```python
from build123d import *

# Parameters (mm, degrees)
SKETCH1_W           = 12.45
SKETCH1_H           = 21.45
BOSS_EXTRUDE1_DEPTH = 18
SKETCH2_W           = 10
SKETCH2_H           = 3
BOSS_EXTRUDE2_DEPTH = 18
SKETCH4_W           = 7
SKETCH4_H           = 8.185466936
SKETCH4_H_2         = 9.121133548
SKETCH4_H_3         = 13.415591142
SKETCH4_H_4         = 10.11507115
SKETCH4_H_5         = 8.575799248
CUT_EXTRUDE2_DEPTH  = 6
FILLET3_R           = 3.5
FILLET4_R           = 2
SKETCH5_R           = 1.6
CUT_EXTRUDE3_DEPTH  = 105.163684291
CUT_EXTRUDE4_DEPTH  = 105.163684291
SKETCH10_W          = 7.3675
SKETCH10_H          = 18
SKETCH10_R          = 1.6
BOSS_EXTRUDE4_DEPTH = 21.45
FILLET6_R           = 3
SKETCH11_W          = 114.139507882
SKETCH11_H          = 1
CUT_EXTRUDE5_DEPTH  = 97.285728563
CHAMFER1_SIZE       = 1
CHAMFER2_SIZE       = 1
FILLET7_R           = 1
FILLET8_R           = 1
FILLET9_R           = 1
SKETCH13_R          = 2.05
CUT_EXTRUDE6_DEPTH  = 8
SKETCH14_R          = 2.05
CUT_EXTRUDE7_DEPTH  = 10
SKETCH15_W          = 114.000331722
SKETCH15_H          = 33.1435942
CUT_EXTRUDE9_DEPTH  = 97.285728563


with BuildPart() as part:
    # Sketch1 → Boss-Extrude1 (new body)
    with BuildSketch(Plane(origin=(0, 0, 0), x_dir=(1, 0, 0), z_dir=(0, 1, 0))):
        Polygon((-19.225, -19.625), (-5.1, -19.625), (-5.1, -13.725), (5.1, -13.725), (5.1, -19.625), (14.35, -19.625), (14.35, -13.725), (24.55, -13.725), (24.55, -19.625), (33.8, -19.625), (33.8, -13.725), (44, -13.725), (44, -19.625), (53.25, -19.625), (53.25, -13.725), (63.45, -13.725), (63.45, -19.625), (72.7, -19.625), (72.7, -13.725), (82.9, -13.725), (82.9, -19.625), (97.025, -19.625), (97.025, -10.725), (87.025, -10.725), (87.025, 13.725), (-9.225, 13.725), (-9.225, -10.725), (-19.225, -10.725), align=None)
        Rectangle(SKETCH1_W, SKETCH1_H, mode=Mode.SUBTRACT)
        with Locations((19.45, 0)):
            Rectangle(SKETCH1_W, SKETCH1_H, mode=Mode.SUBTRACT)
        with Locations((38.9, 0)):
            Rectangle(SKETCH1_W, SKETCH1_H, mode=Mode.SUBTRACT)
        with Locations((58.35, 0)):
            Rectangle(SKETCH1_W, SKETCH1_H, mode=Mode.SUBTRACT)
        with Locations((77.8, 0)):
            Rectangle(SKETCH1_W, SKETCH1_H, mode=Mode.SUBTRACT)
    extrude(amount=BOSS_EXTRUDE1_DEPTH)

    # Sketch2 → Boss-Extrude2 (add)
    with BuildSketch(Plane(origin=(0, 18, 0), x_dir=(1, 0, 0), z_dir=(0, 1, 0))):
        with Locations((-14.225, -9.225)):
            Rectangle(SKETCH2_W, SKETCH2_H)
        with Locations((92.025, -9.225)):
            Rectangle(SKETCH2_W, SKETCH2_H)
    extrude(amount=-BOSS_EXTRUDE2_DEPTH)

    # Sketch4 → Cut-Extrude2 (cut)
    with BuildSketch(Plane(origin=(0, 18, 0), x_dir=(1, 0, 0), z_dir=(0, 1, 0))):
        with Locations((0, 10.725)):
            Rectangle(SKETCH4_W, SKETCH4_H)
        with Locations((19.45, 10.725)):
            Rectangle(SKETCH4_W, SKETCH4_H_2)
        with Locations((38.9, 10.725)):
            Rectangle(SKETCH4_W, SKETCH4_H_3)
        with Locations((58.35, 10.725)):
            Rectangle(SKETCH4_W, SKETCH4_H_4)
        with Locations((77.8, 10.725)):
            Rectangle(SKETCH4_W, SKETCH4_H_5)
    extrude(amount=-CUT_EXTRUDE2_DEPTH, mode=Mode.SUBTRACT)

    # Fillet3
    fillet3_edges = [part.edges().sort_by_distance(p)[0] for p in [
        (81.3, 12, -12.225),
        (74.3, 12, -12.225),
        (54.85, 12, -12.225),
        (61.85, 12, -12.225),
        (42.4, 12, -12.225),
        (35.4, 12, -12.225),
        (15.95, 12, -12.225),
        (22.95, 12, -12.225),
        (3.5, 12, -12.225),
        (-3.5, 12, -12.225),
    ]]
    fillet(fillet3_edges, radius=FILLET3_R - 0.0001)  # a hair under: the kernel refuses the full size

    # Fillet4
    fillet4_edges = [part.edges().sort_by_distance(p)[0] for p in [
        (74.3, 18, -12.225),
        (81.3, 18, -12.225),
        (54.85, 18, -12.225),
        (61.85, 18, -12.225),
        (35.4, 18, -12.225),
        (42.4, 18, -12.225),
        (15.95, 18, -12.225),
        (22.95, 18, -12.225),
        (-3.5, 18, -12.225),
        (3.5, 18, -12.225),
    ]]
    fillet(fillet4_edges, radius=FILLET4_R)

    # Sketch5 → Cut-Extrude3 (cut, through all)
    with BuildSketch(Plane.XY.offset(19.625)):
        with Locations((9.725, 9)):
            Circle(SKETCH5_R)
        with Locations((29.175, 9)):
            Circle(SKETCH5_R)
        with Locations((48.625, 9)):
            Circle(SKETCH5_R)
        with Locations((68.075, 9)):
            Circle(SKETCH5_R)
        with Locations((87.53, 9)):
            Circle(SKETCH5_R)
        with Locations((-9.73, 9)):
            Circle(SKETCH5_R)
    extrude(amount=-CUT_EXTRUDE3_DEPTH, mode=Mode.SUBTRACT)

    # Sketch7 → Cut-Extrude4 (cut, through all)
    with BuildSketch(Plane(origin=(0, 0, -13.725), x_dir=(-1, 0, 0), z_dir=(0, 0, -1))):
        Polygon((-92.53, 9), (-92.53, -2.934603673), (-102.870987394, -2.934603673), (-102.870987394, 21.319522162), (-92.53, 21.319522162), align=None)
        Polygon((14.73, 9), (14.73, -3.337317556), (26.94038456, -3.337317556), (26.94038456, 20.180651888), (14.73, 20.180651888), align=None)
    extrude(amount=-CUT_EXTRUDE4_DEPTH, mode=Mode.SUBTRACT)

    # Sketch10 → Boss-Extrude4 (add)
    # profile 1 of 2: a face of its own
    with BuildSketch(Plane(origin=(0, 0, 7.725), x_dir=(-1, 0, 0), z_dir=(0, 0, -1))):
        with Locations((-88.84625, 9)):
            Rectangle(SKETCH10_W, SKETCH10_H)
        with Locations(Location((-87.53, 9, 0), (0, 0, 180))):
            Circle(SKETCH10_R, mode=Mode.SUBTRACT)
    # profile 2 of 2: a face of its own
    with BuildSketch(Plane(origin=(0, 0, 7.725), x_dir=(-1, 0, 0), z_dir=(0, 0, -1))):
        with Locations((11.04625, 9)):
            Rectangle(SKETCH10_W, SKETCH10_H)
        with Locations(Location((9.73, 9, 0), (0, 0, 180))):
            Circle(SKETCH10_R, mode=Mode.SUBTRACT)
    extrude(amount=BOSS_EXTRUDE4_DEPTH)

    # Fillet6
    fillet6_edges = [part.edges().sort_by_distance(p)[0] for p in [
        (92.53, 18, 2.95),
        (-14.73, 18, 2.95),
    ]]
    fillet(fillet6_edges, radius=FILLET6_R)

    # Sketch11 → Cut-Extrude5 (cut, through all)
    with BuildSketch(Plane(origin=(0, 18, 0), x_dir=(1, 0, 0), z_dir=(0, 1, 0))):
        with Locations((38.937615411, 5.225)):
            Rectangle(SKETCH11_W, SKETCH11_H)
    extrude(amount=-CUT_EXTRUDE5_DEPTH, mode=Mode.SUBTRACT)


with BuildPart() as cut_extrude5_piece_1:
    # of the separate pieces the step leaves, piece 1, a body of its own (cut_extrude5_pieces)
    add(part.part.solids().sort_by_distance((-11.73, 18, -4.725))[0])

    # Chamfer2
    chamfer2_edges = [cut_extrude5_piece_1.edges().sort_by_distance(p)[0] for p in [
        (-9.915, 0, 19.625),
        (-14.73, 0, 7.45),
        (68.075, 0, 19.625),
        (63.45, 0, 16.675),
        (58.35, 0, 13.725),
        (53.25, 0, 16.675),
        (48.625, 0, 19.625),
        (44, 0, 16.675),
        (38.9, 0, 13.725),
        (33.8, 0, 16.675),
        (29.175, 0, 19.625),
        (24.55, 0, 16.675),
        (19.45, 0, 13.725),
        (14.35, 0, 16.675),
        (9.725, 0, 19.625),
        (5.1, 0, 16.675),
        (0, 0, 13.725),
        (-5.1, 0, 16.675),
        (92.53, 0, 7.45),
        (-6.225, 0, 3),
        (6.225, 0, 3),
        (25.675, 0, 3),
        (87.715, 0, 19.625),
        (13.225, 0, 3),
        (45.125, 0, 3),
        (32.675, 0, 3),
        (64.575, 0, 3),
        (52.125, 0, 3),
        (84.025, 0, 3),
        (71.575, 0, 3),
        (82.9, 0, 16.675),
        (77.8, 0, 13.725),
        (72.7, 0, 16.675),
        (77.8, 0, 10.725),
        (9.725, 0, -4.725),
        (88.2775, 0, -4.725),
        (68.075, 0, -4.725),
        (48.625, 0, -4.725),
        (29.175, 0, -4.725),
        (-10.4775, 0, -4.725),
        (58.35, 0, 10.725),
        (38.9, 0, 10.725),
        (19.45, 0, 10.725),
        (0, 0, 10.725),
    ]]
    chamfer(chamfer2_edges, length=CHAMFER2_SIZE)

    # Fillet7
    fillet7_edges = [cut_extrude5_piece_1.edges().sort_by_distance(p)[0] for p in [
        (91.651320344, 17.121320344, -4.725),
        (71.575, 9.5, -4.725),
        (52.125, 9.5, -4.725),
        (32.675, 9.5, -4.725),
        (13.225, 9.5, -4.725),
        (6.225, 9.5, -4.725),
        (84.025, 9.5, -4.725),
        (64.575, 9.5, -4.725),
        (45.125, 9.5, -4.725),
        (25.675, 9.5, -4.725),
        (-6.225, 9.5, -4.725),
        (-14.73, 8, -4.725),
        (-13.851320344, 17.121320344, -4.725),
        (9.725, 18, -4.725),
        (86.7775, 18, -4.725),
        (68.075, 18, -4.725),
        (48.625, 18, -4.725),
        (29.175, 18, -4.725),
        (-8.9775, 18, -4.725),
        (92.53, 8, -4.725),
    ]]
    fillet(fillet7_edges, radius=FILLET7_R)

    # Sketch13 → Cut-Extrude6 (cut)
    with BuildSketch(Plane.XY.offset(19.625)):
        with Locations((-9.73, 9)):
            Circle(SKETCH13_R)
        with Locations((9.725, 9)):
            Circle(SKETCH13_R)
        with Locations((29.175, 9)):
            Circle(SKETCH13_R)
        with Locations((48.625, 9)):
            Circle(SKETCH13_R)
        with Locations((68.075, 9)):
            Circle(SKETCH13_R)
        with Locations((87.53, 9)):
            Circle(SKETCH13_R)
    extrude(amount=-CUT_EXTRUDE6_DEPTH, mode=Mode.SUBTRACT)

    # Sketch14 → Cut-Extrude7 (cut)
    with BuildSketch(Plane(origin=(0, 0, -4.725), x_dir=(-1, 0, 0), z_dir=(0, 0, -1))):
        with Locations(Location((-87.53, 9, 0), (0, 0, 180))):
            Circle(SKETCH14_R)
        with Locations(Location((-68.075, 9, 0), (0, 0, 180))):
            Circle(SKETCH14_R)
        with Locations(Location((-48.625, 9, 0), (0, 0, 180))):
            Circle(SKETCH14_R)
        with Locations(Location((-29.175, 9, 0), (0, 0, 180))):
            Circle(SKETCH14_R)
        with Locations(Location((-9.725, 9, 0), (0, 0, 180))):
            Circle(SKETCH14_R)
        with Locations(Location((9.73, 9, 0), (0, 0, 180))):
            Circle(SKETCH14_R)
    extrude(amount=-CUT_EXTRUDE7_DEPTH, mode=Mode.SUBTRACT)


with BuildPart() as cut_extrude5_piece_2:
    # of the separate pieces the step leaves, piece 2, a body of its own (cut_extrude5_pieces)
    add(part.part.solids().sort_by_distance((-11.73, 18, -13.725))[0])

    # Chamfer1
    chamfer1_edges = [cut_extrude5_piece_2.edges().sort_by_distance(p)[0] for p in [
        (77.8, 0, -10.725),
        (58.35, 0, -10.725),
        (38.9, 0, -10.725),
        (6.225, 0, -8.225),
        (19.45, 0, -10.725),
        (0, 0, -10.725),
        (84.025, 0, -8.225),
        (64.575, 0, -8.225),
        (45.125, 0, -8.225),
        (25.675, 0, -8.225),
        (92.53, 0, -9.725),
        (88.2775, 0, -5.725),
        (71.575, 0, -8.225),
        (68.075, 0, -5.725),
        (52.125, 0, -8.225),
        (48.625, 0, -5.725),
        (32.675, 0, -8.225),
        (29.175, 0, -5.725),
        (13.225, 0, -8.225),
        (9.725, 0, -5.725),
        (-6.225, 0, -8.225),
        (-10.4775, 0, -5.725),
        (-14.73, 0, -9.725),
        (38.9, 0, -13.725),
    ]]
    chamfer(chamfer1_edges, length=CHAMFER1_SIZE)

    # Fillet8
    fillet8_edges = [cut_extrude5_piece_2.edges().sort_by_distance(p)[0] for p in [
        (-14.73, 8, -5.725),
        (-6.225, 9.5, -5.725),
        (6.225, 9.5, -5.725),
        (13.225, 9.5, -5.725),
        (25.675, 9.5, -5.725),
        (32.675, 9.5, -5.725),
        (45.125, 9.5, -5.725),
        (52.125, 9.5, -5.725),
        (64.575, 9.5, -5.725),
        (71.575, 9.5, -5.725),
        (84.025, 9.5, -5.725),
        (91.651320344, 17.121320344, -5.725),
        (86.7775, 18, -5.725),
        (-8.9775, 18, -5.725),
        (-13.851320344, 17.121320344, -5.725),
        (9.725, 18, -5.725),
        (29.175, 18, -5.725),
        (48.625, 18, -5.725),
        (68.075, 18, -5.725),
        (92.53, 8, -5.725),
    ]]
    fillet(fillet8_edges, radius=FILLET8_R)

    # Fillet9
    fillet9_edges = [cut_extrude5_piece_2.edges().sort_by_distance(p)[0] for p in [
        (-2.474903023, 13.025096977, -13.725),
        (2.474903023, 13.025096977, -13.725),
        (4.085786438, 17.414213562, -13.725),
        (9.725, 18, -13.725),
        (15.364213562, 17.414213562, -13.725),
        (16.975096977, 13.025096977, -13.725),
        (21.924903023, 13.025096977, -13.725),
        (23.535786438, 17.414213562, -13.725),
        (29.175, 18, -13.725),
        (34.814213562, 17.414213562, -13.725),
        (36.425096977, 13.025096977, -13.725),
        (41.374903023, 13.025096977, -13.725),
        (42.985786438, 17.414213562, -13.725),
        (48.625, 18, -13.725),
        (54.264213562, 17.414213562, -13.725),
        (55.875096977, 13.025096977, -13.725),
        (60.824903023, 13.025096977, -13.725),
        (62.435786438, 17.414213562, -13.725),
        (68.075, 18, -13.725),
        (73.714213562, 17.414213562, -13.725),
        (75.325096977, 13.025096977, -13.725),
        (80.274903023, 13.025096977, -13.725),
        (81.885786438, 17.414213562, -13.725),
        (86.415, 18, -13.725),
        (91.651320344, 17.121320344, -13.725),
        (92.53, 8, -13.725),
        (-14.73, 8, -13.725),
        (81.3, 15.74995, -13.725),
        (74.3, 15.74995, -13.725),
        (61.85, 15.74995, -13.725),
        (54.85, 15.74995, -13.725),
        (42.4, 15.74995, -13.725),
        (35.4, 15.74995, -13.725),
        (22.95, 15.74995, -13.725),
        (15.95, 15.74995, -13.725),
        (3.5, 15.74995, -13.725),
        (-3.5, 15.74995, -13.725),
        (-13.851320344, 17.121320344, -13.725),
        (-8.615, 18, -13.725),
        (-4.085786438, 17.414213562, -13.725),
    ]]
    fillet(fillet9_edges, radius=FILLET9_R)

    # Sketch15 → Cut-Extrude9 (cut, through all)
    with BuildSketch(Plane.XZ):
        with Locations((36.723202727, -21.801193098)):
            Rectangle(SKETCH15_W, SKETCH15_H)
    extrude(amount=-CUT_EXTRUDE9_DEPTH, mode=Mode.SUBTRACT)


solid = cut_extrude5_piece_1.part
```
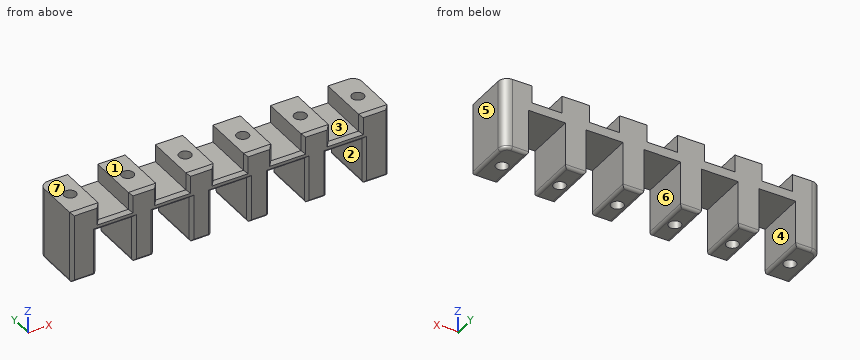
Geometry: final body of the model. Coordinates: model frame, mm. Face numbers are marked on the shaded views. A direction names the side the tool comes from. Coordinates: 2 decimals unless noted, no trailing zeros. Order: outer loops, then holes, each group sorted by start corner. A loop starts at its lowest first (then second) coordinate and runs counter-clockwise, first axis right, second up. Notation, with made-up numbers: (77, 41) - (102, 41) arc R20 ccw to (102, 55) - close; hole circle Ø5 at (-37, -39). An arc over 180 degrees is marked (long way). Write each question's results on one line, items separated by ' | '.
(1) First-contact query: pin 1 Ø5 at (x, y) = (56.5, 14) entering from -Z (3 decimals); pin 2 Ø4.5 at (x, y) = (28.5, 10) entering from -Z (3 decimals); pin 3 Ø3.5 at (x, y) = (9.725, 9) entering from +Z (3 decimals); pin 4 Ø8 at (x, z) = (76.5, 7.5) entering from -Y (3 decimals). Flat tips, straight axial feed; report the tip coordinate or a pass-through.
Values found:
pin 1: stops at z = 10.725 | pin 2: stops at z = -4.725 | pin 3: stops at z = 11.625 | pin 4: stops at y = 0.225
(2) Set-up query: the marked faces 1, 2 and 3. Return all of +Z, -Z, +X, -X, +Y, -Y with unobstructed straight access to the full face (end or side cutting, diameter ignored); none if empty.
Values found:
face 1: +Z, +X, -X, +Y, -Y | face 2: -Z, +Y, -Y | face 3: +Z, +Y, -Y
(3) Section query A-A, the plane x = 87.53. Return the cut outline in (y, z) (3 decimals).
Values found:
outline: (0, -3.725) - (1, -4.725) - (6.95, -4.725) - (6.95, 5.275) - (7.4, 5.275) - (7.4, 11.625) - (6.95, 11.625) - (6.95, 19.625) - (1, 19.625) - (0, 18.625) - close; (10.6, 5.275) - (11.05, 5.275) - (11.05, -4.725) - (17, -4.725) arc R1 ccw to (18, -3.725) - (18, 19.625) - (11.05, 19.625) - (11.05, 11.625) - (10.6, 11.625) - close
(4) Line query: line 1 (X direction, y = 1.5, z = 8.75) (3 decimals); line 2 (X direction, y = 17, z = 5.25) (3 decimals); line 3 (Y direction, x = 87.53, z = 9.75). Output: solid intervals per line, ascending. Write a range as [from, to].
Values found:
line 1: x = [-14.73, -6.225], [6.225, 13.225], [25.675, 32.675], [45.125, 52.125], [64.575, 71.575], [84.025, 92.53] | line 2: x = [-13.966, -6.225], [6.225, 13.225], [25.675, 32.675], [45.125, 52.125], [64.575, 71.575], [84.025, 91.766] | line 3: y = [0, 7.4], [10.6, 18]
(5) Section query D-D, the plane x = 59. Return the cut outline in (y, z) (3 decimals), plus the area to 3 significant figures.
Values found:
outline: (0, 11.725) - (1, 10.725) - (18, 10.725) - (18, 13.725) - (1, 13.725) - (0, 12.725) - close | area: 53.0 mm²
(6) Section query B-B, the plane z = 3.5. Count the separate pieces of the cut face and the enclosed holes in it, plus the area to 3 significant figures.
Values found:
separate pieces: 6 | enclosed holes: 6 | area: 721 mm²
(7) Mould query, pull axis X, two halves, no side actions, for the marked faces 4, 5, 6 and 7. Classes: +X half, -X half, draft (parallel to the pull), parting line (faces both ways), or undercut.
Values found:
face 4: undercut | face 5: +X half | face 6: undercut | face 7: draft
